For this review, take the finished solid that the model builds, in its own axes (mm). Face numbers are marked on the shaded views. A direction names the side the tool comes from. Round coordinates to 2 decimals unless told otherwise and drop trailing zeros. Order: outer loops, then holes, each group sorted by start corner. A loop starts at its lowest first (then second) coordinate and runs counter-clockwise, first axis right, second up. Notation, with made-up numbers: (74.25, 15.5) - (123.25, 15.5) arc R27 cw to (123.25, 33.5) - close; hole circle Ø7 at (54.5, -6). An arc over 180 degrees is marked (long way). Write each question's results on one line, items separated by ' | '. Start each with the question number.
(1) Take a section at A-A, the plane y = 6. Give the boundary of the cut face in (x, z).
(2) For L1, parallel to Y at x = 10, z = -4.3; L2, parallel to Y at x = -15, z = -7.75; L3, parallel to X at y = -4.5, z = -12.5, list the stretches that pass through material, from the lowest coordinate up. Write a range as from..to.
(3) For the marked faces 4, 5 and 6, list the 3-axis set-ups (+Z, -Z, +X, -X, +Y, -Y) from which the entire face can be reached by the end or side of a thin tool; tool diameter is ignored.
(4) Take a section at C-C, the plane y = 13.5. Give the boundary of the cut face in (x, z), plus the area to 3 significant figures.
(5) Draft analysis for pull direction Y (two halves, no side actions). For the marked faces 1, 2 and 3, state which applies: pulls with the +Y half, pulls with the -Y half, needs draft (parallel to the pull), parting line crosses it, or undercut.
(6) Insertion check: pin 1 Ø6 at (x, z) = (-5, -19.5) entering from +Y; pin 2 Ø6 at (x, z) = (11, -16.5) entering from -Y; pin 3 Ø5 at (x, y) = (-10, 6) entering from -Z. Each pin has a flat end and moves straight along its axis. Give the tip position at first contact, or say it passes through.
(7) Take a section at B-B, the plane x = -10. Give the boundary of the cut face in (y, z), plus the area to 3 significant figures.
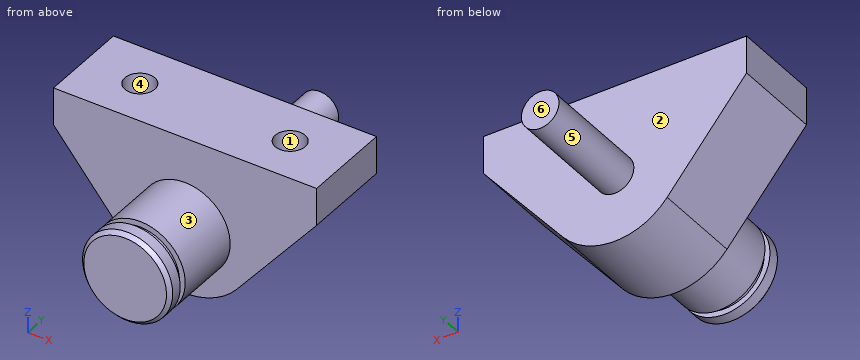
```python
from build123d import *

# Parameters (mm, degrees)
EXTRUDE_1_DEPTH     = 12
SKETCH_2_R          = 6
EXTRUDE_2_DEPTH     = 9
SKETCH_3_R          = 5.25
EXTRUDE_3_DEPTH     = 1
SKETCH_4_R          = 6
EXTRUDE_4_DEPTH     = 2
CHAMFER_1_SIZE      = 0.5
SKETCH_5_R          = 2
CUT_EXTRUDE_1_DEPTH = 5
SKETCH_6_R          = 2.5
EXTRUDE_5_DEPTH     = 15


with BuildPart() as part:
    # 草图1 → 凸台-拉伸1 (new body)
    with BuildSketch(Plane(origin=(0, 0, 0), x_dir=(1, 0, 0), z_dir=(0, 1, 0))):
        with BuildLine():
            Line((-17.5, 6.09769995), (-6.926984364, 18.843732288))
            ThreePointArc((-6.926984364, 18.843732288), (0, 22.09769995), (6.926984364, 18.843732288))
            Line((6.926984364, 18.843732288), (17.5, 6.09769995))
            Line((17.5, 6.09769995), (17.5, 1.09769995))
            Line((17.5, 1.09769995), (-17.5, 1.09769995))
            Line((-17.5, 1.09769995), (-17.5, 6.09769995))
        make_face()
    extrude(amount=EXTRUDE_1_DEPTH)

    # 草图2 → 凸台-拉伸2 (add)
    with BuildSketch(Plane(origin=(0, 0, 0), x_dir=(1, 0, 0), z_dir=(0, 1, 0))):
        with Locations(Location((0, 13.09769995, 0), (0, 0, 270))):
            Circle(SKETCH_2_R)
    extrude(amount=-EXTRUDE_2_DEPTH)

    # 草图3 → 凸台-拉伸3 (add)
    with BuildSketch(Plane(origin=(0, -9, 0), x_dir=(-1, 0, 0), z_dir=(0, -1, 0))):
        with Locations(Location((0, 13.09769995, 0), (0, 0, 270))):
            Circle(SKETCH_3_R)
    extrude(amount=EXTRUDE_3_DEPTH)

    # 草图4 → 凸台-拉伸4 (add)
    with BuildSketch(Plane(origin=(0, -10, 0), x_dir=(-1, 0, 0), z_dir=(0, -1, 0))):
        with Locations(Location((0, 13.09769995, 0), (0, 0, 270))):
            Circle(SKETCH_4_R)
    extrude(amount=EXTRUDE_4_DEPTH)

    # 倒角1
    chamfer_1_edges = [part.edges().sort_by_distance(p)[0] for p in [
        (0, -12, -19.09769995),
    ]]
    chamfer(chamfer_1_edges, length=CHAMFER_1_SIZE)

    # 草图5 → 切除-拉伸1 (cut)
    with BuildSketch(Plane.XY.offset(-1.09769995)):
        with Locations((-10, 6)):
            Circle(SKETCH_5_R)
        with Locations(Location((10, 6, 0), (0, 0, 180))):
            Circle(SKETCH_5_R)
    extrude(amount=-CUT_EXTRUDE_1_DEPTH, mode=Mode.SUBTRACT)

    # 草图6 → 凸台-拉伸5 (add)
    with BuildSketch(Plane(origin=(0, 12, 0), x_dir=(1, 0, 0), z_dir=(0, 1, 0))):
        with Locations(Location((0, 13.09769995, 0), (0, 0, 90))):
            Circle(SKETCH_6_R)
    extrude(amount=EXTRUDE_5_DEPTH)


solid = part.part
```
Results below:
1) outline: (-17.5, -6.1) - (-6.93, -18.84) arc R9 ccw to (6.93, -18.84) - (17.5, -6.1) - (17.5, -1.1) - (12, -1.1) - (12, -6.1) - (8, -6.1) - (8, -1.1) - (-8, -1.1) - (-8, -6.1) - (-12, -6.1) - (-12, -1.1) - (-17.5, -1.1) - close
2) L1: y = 0..4, 8..12 | L2: y = 0..12 | L3: x = -5.97..5.97
3) face 4: +Z | face 5: +Y | face 6: +Z, -Z, +X, -X, +Y
4) outline: circle Ø5 at (0, -13.1) | area: 19.6 mm^2
5) face 1: undercut | face 2: pulls with the +Y half | face 3: needs draft
6) pin 1: stops at y = 12 | pin 2: stops at y = 0 | pin 3: stops at z = -18.15
7) outline: (0, -15.14) - (12, -15.14) - (12, -1.1) - (8, -1.1) - (8, -6.1) - (4, -6.1) - (4, -1.1) - (0, -1.1) - close | area: 148 mm^2
